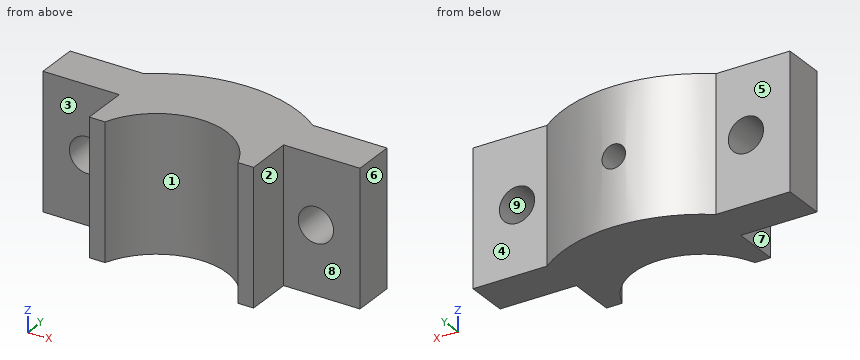
from build123d import *

# Parameters (mm, degrees)
BOSS_EXTRUDE1_DEPTH  = 23
SKETCH2_R            = 6
CUT_EXTRUDE1_DEPTH   = 67.104489714
CUT_EXTRUDE2_START   = -8.577540152
CUT_EXTRUDE2_DEPTH   = 19.577540152
CUT_EXTRUDE2_START_2 = -5
CUT_EXTRUDE2_2_DEPTH = 10


with BuildPart() as part:
    # Sketch1 → Boss-Extrude1 (new, symmetric)
    with BuildSketch(Plane.XY):
        with BuildLine():
            Line((-22.627416998, 8), (-28, 8))
            Line((-28, 8), (-28, 24))
            Line((-28, 24), (-54, 24))
            Line((-54, 24), (-54, 38.410583031))
            Line((-54, 38.410583031), (-28.785883888, 38.410583031))
            ThreePointArc((-28.785883888, 38.410583031), (0, 48), (28.785883888, 38.410583031))
            Line((28.785883888, 38.410583031), (54, 38.410583031))
            Line((54, 38.410583031), (54, 24))
            Line((54, 24), (28, 24))
            Line((28, 24), (28, 8))
            Line((28, 8), (22.627416998, 8))
            ThreePointArc((22.627416998, 8), (0, 24), (-22.627416998, 8))
        make_face()
    extrude(amount=BOSS_EXTRUDE1_DEPTH, both=True)

    # Sketch2 → Cut-Extrude1 (cut, through all)
    with BuildSketch(Plane(origin=(0, 38.410583031, 0), x_dir=(1, 0, 0), z_dir=(0, 1, 0))):
        with Locations(Location((-39, 0, 0), (0, 0, 270))):
            Circle(SKETCH2_R)
        with Locations(Location((39, 0, 0), (0, 0, 270))):
            Circle(SKETCH2_R)
    extrude(amount=-CUT_EXTRUDE1_DEPTH, mode=Mode.SUBTRACT)

    # Cut-Extrude2: read off the stored shape, not the designer's step
    # Cut-Extrude2 outline → Cut-Extrude2 (cut)
    with BuildSketch(Plane(origin=(0, 38.410583031, 0), x_dir=(1, 0, 0), z_dir=(0, 1, 0)).offset(CUT_EXTRUDE2_START)):
        with BuildLine():
            add(Edge.make_bspline(
                [(0, 4), (-1.057527997, 4), (-2.091087742, 3.565911724), (-3.566323367, 2.090385612), (-3.999433765, 1.046115956), (-4.00056506, -1.04178128), (-3.576219278, -2.07994956), (-2.083227921, -3.574310552), (-1.045821073, -3.9996204), (1.042915307, -4.000379072), (2.087446575, -3.567981834), (3.563947107, -2.094327717), (3.998968512, -1.060310778), (4.001027689, 1.052513916), (3.568016054, 2.087668509), (2.093312914, 3.564707479), (1.057527997, 4), (0, 4)],
                knots=[0, 0, 0, 0, 0.125, 0.125, 0.25, 0.25, 0.375, 0.375, 0.5, 0.5, 0.625, 0.625, 0.75, 0.75, 0.875, 0.875, 1, 1, 1, 1], degree=3))
        make_face()
    extrude(amount=CUT_EXTRUDE2_DEPTH, mode=Mode.SUBTRACT)

    # Cut-Extrude2 2 outline → Cut-Extrude2 2 (add)
    with BuildSketch(Plane.XY.offset(CUT_EXTRUDE2_START_2)):
        with BuildLine():
            ThreePointArc((4.00000004, 29.83304297), (-2.3e-08, 30), (-4.000000085, 29.833042966))
            Line((-4.000000085, 29.833042966), (4.00000004, 29.83304297))
        make_face()
    extrude(amount=CUT_EXTRUDE2_2_DEPTH)


solid = part.part
Could you check a few things on this model? Use its own coordinates, in mm. Face numbers are marked on the shaded views. A direction names the side the tool comes from. Coordinates: 2 decimals unless noted, no trailing zeros. Write each loop counter-clockwise with the first axis right and the second up, starting at its lowest first coordinate (ties: lowest second). Pieces come first, ordered by that corner, then holes. Notation, with made-up numbers: (81, -29) - (129, -29) arc R18 cw to (129, 4) - close; hole circle Ø2 at (2, 54.25). An arc over 180 degrees is marked (long way). Put each result on its own line as item: value. Start each with the question number.
Q1. I want a section at D-D on y = 32.5. Count the separate pieces of the cut face and the enclosed holes in it, plus the area to 3 significant figures.
Q2. I want a section at A-A on x = 39. Write out the boundary of the cut face in (y, z), plus the area to 3 significant figures.
Q3. I'm going to push flat-ended pins straight in: P1, Ø8, axis at x = -42, z = 5, coming from the -Y side; P2, Ø10, axis at x = -24.5, z = 0.5, coming from the +Y side; P3, Ø4, axis at y = 18.5, z = 3.5, coming from the +X side. Where does each tip first touch, or does it pass through?
Q4. Thinking about a two-plate mould opening in X: for the marked faces 6, 7, 8 and 9, which applies, pulls with the +X half, pulls with the -X half, needs draft (parallel to the pull), parting line crosses it, or undercut?
Q5. Which directions (+Z, -Z, +X, -X, +Y, -Y) give clear straight access to the entire face, cutting with the end or side of a thin tool? Please do the marked faces 1, 2, 3, 4 and 5.
Q6. I want a section at C-C on z = 19.5. Write out the boundary of the cut face in (x, y).
Q7. I want a section at B-B on y = 19.5. Write out the boundary of the cut face in (x, z), plus the area to 3 significant figures.
Q8. Please list where these lines run through material, in increasing order: L1, parallel to X at y = 29, z = 0; L2, parallel to X at y = 32, z = 0; L3, parallel to X at y = 39, z = 10.
Checks:
1. separate pieces: 1
1. enclosed holes: 3
1. area: 4,690 mm²
2. outline: (24, -23) - (38.41, -23) - (38.41, -6) - (24, -6) - close; (24, 6) - (38.41, 6) - (38.41, 23) - (24, 23) - close
2. area: 490 mm²
3. P1: y = 24
3. P2: y = 43.86
3. P3: x = 28
4. face 6: pulls with the +X half
4. face 7: pulls with the -X half
4. face 8: needs draft
4. face 9: undercut
5. face 1: +Z, -Z, -Y
5. face 2: +Z, -Z, +X, -Y
5. face 3: +Z, -Z, -X, -Y
5. face 4: +Z, -Z, +X, +Y
5. face 5: +Z, -Z, -X, +Y
6. outline: (-54, 24) - (-28, 24) - (-28, 8) - (-22.63, 8) arc R24 cw to (22.63, 8) - (28, 8) - (28, 24) - (54, 24) - (54, 38.41) - (28.79, 38.41) arc R48 ccw to (-28.79, 38.41) - (-54, 38.41) - close
7. outline: (-28, -23) - (-13.99, -23) - (-13.99, 23) - (-28, 23) - close; (13.99, -23) - (28, -23) - (28, 23) - (13.99, 23) - close
7. area: 1,290 mm²
8. L1: -54 to -45, -33 to 33, 45 to 54
8. L2: -54 to -45, -33 to -4, 4 to 33, 45 to 54
8. L3: -27.98 to 27.98
